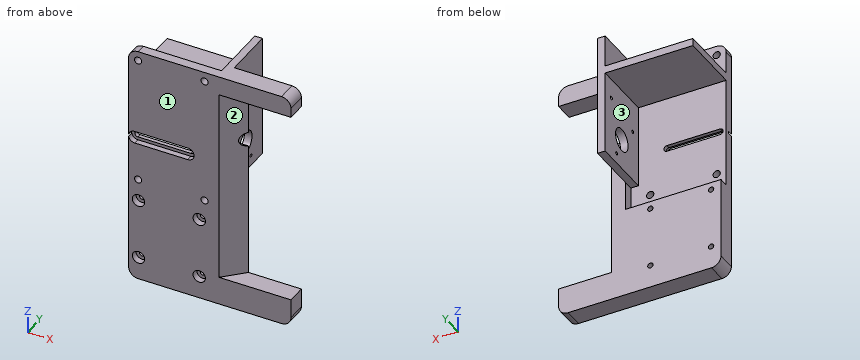
Autodesk Inventor part; units mm, degrees
ref_plane "Arbeitsebene4" through (-41.55, 10, -74.35) normal (0, -1, 0) x (1, 0, 0)
ref_plane "Arbeitsebene5" through (-44.55, 5, -0.85) normal (0, -1, 0) x (1, 0, 0)
ref_plane "Arbeitsebene7" through (7.45, -0.1921, -3.518) normal (-1, 0, 0) x (0, -0.417504, 0.9086751)
ref_plane "Arbeitsebene4" through (-41.55, 10, -74.35) normal (0, -1, 0) x (1, 0, 0)
sketch "Skizze1" plane through (0, 0, 0) normal (0, 1, 0) x (-1, 0, 0)
  line L0 (-37.75, -63.9) -> (37.75, -63.9)
  line L1 (42.75, -58.9) -> (42.75, 58.9)
  line L2 (37.75, 63.9) -> (-37.75, 63.9)
  line L3 (-42.75, 58.9) -> (-42.75, -58.9)
  line L4 (-42.75, -63.9) -> (42.75, 63.9) construction
  line L5 (42.75, -63.9) -> (-42.75, 63.9) construction
  arc A0 (42.75, 58.9) -> (37.75, 63.9) centre (37.75, 58.9) ccw
  arc A1 (-37.75, 63.9) -> (-42.75, 58.9) centre (-37.75, 58.9) ccw
  arc A2 (-42.75, -58.9) -> (-37.75, -63.9) centre (-37.75, -58.9) ccw
  arc A3 (37.75, -63.9) -> (42.75, -58.9) centre (37.75, -58.9) ccw
  point P0 (0, 0)
  dimension "d0" = 85.5
  dimension "d1" = 127.8
  dimension "d2" = 5
extrude "Extrusion1" add sketch "Skizze1" along normal up to surface (10 mm away)
ref_plane "Arbeitsebene1" through (37.75, 0, 0) normal (0, 0, -1) x (-1, 0, 0)
ref_plane "Arbeitsebene2" through (0, 0, 58.9) normal (1, 0, 0) x (0, 0, -1)
sketch "Skizze10" plane through (0, 0, 0) normal (0, -1, 0) x (1, 0, 0)
  circle A0 centre (-37.55, -51.85) radius 1.75
  circle A1 centre (-37.55, -19.85) radius 1.75
  circle A2 centre (-5.55, -51.85) radius 1.75
  circle A3 centre (-5.55, -19.85) radius 1.75
  circle A4 centre (-37.55, -51.85) radius 1.4
  point P0 (0, 0)
  dimension "d37" = 2.8
hole "Bohrung2" at (-37.55, 0, -51.85) at (-37.55, 0, -19.85) at (-5.55, 0, -19.85) at (-5.55, 0, -51.85) direction (0, 1, 0) diameter 2.8 end through all counterbore diameter 6.5 counterbore depth 3.5
sketch "Skizze11" plane through (-37.75, 10, -63.9) normal (0, 1, 0) x (1, 0, 0)
  line L0 (-6.8, -63.05) -> (41.2, -63.05)
  line L1 (-6.8, -95.05) -> (41.2, -95.05)
  line L2 (-3.8, -48.05) -> (36.2, -48.05)
  line L3 (-5, -5) -> (-5, -122.8)
  line L4 (0, -127.8) -> (75.5, -127.8)
  line L5 (-5, -48.05) -> (45.2, -48.05)
  line L6 (45.2, -48.05) -> (45.2, -127.8)
  line L7 (45.2, -127.8) -> (-5, -127.8)
  line L8 (-5, -127.8) -> (-5, -48.05)
  line L9 (45.2, -108.7984) -> (45.2, -60.5539)
  line L10 (80.5, -82.3) -> (60.5, -82.3) construction
  line L11 (60.5, -82.3) -> (60.5, -82.05) construction
  line L12 (60.5, -82.05) -> (60.5, -81.8) construction
  line L13 (60.5, -81.8) -> (60.5, -81.55) construction
  line L14 (60.5, -81.55) -> (60.5, -81.3) construction
  line L15 (60.5, -81.3) -> (60.5, -81.05) construction
  line L16 (60.5, -81.05) -> (60.5, -80.8) construction
  line L17 (60.5, -80.8) -> (60.5, -80.55) construction
  line L18 (60.5, -80.55) -> (60.5, -80.3) construction
  line L19 (60.5, -80.3) -> (60.5, -80.05) construction
  line L20 (60.5, -80.05) -> (60.5, -79.8) construction
  line L21 (60.5, -79.8) -> (60.5, -79.55) construction
  line L22 (60.5, -79.55) -> (60.5, -79.3) construction
  line L23 (60.5, -79.3) -> (60.5, -79.05) construction
  line L24 (60.5, -79.05) -> (60.5, -78.8) construction
  line L25 (60.5, -78.8) -> (60.5, -78.55) construction
  line L26 (60.5, -78.55) -> (60.5, -78.3) construction
  line L27 (60.5, -78.3) -> (60.5, -78.05) construction
  line L28 (60.5, -78.05) -> (60.5, -77.8) construction
  line L29 (60.5, -77.8) -> (60.5, -77.55) construction
  line L30 (60.5, -77.55) -> (60.5, -77.3) construction
  line L31 (60.5, -77.3) -> (80.5, -77.3) construction
  line L32 (80.5, -77.3) -> (80.5, -41.8) construction
  line L33 (80.5, -41.8) -> (54.7, -41.8) construction
  line L34 (54.7, -41.8) -> (54.7, -117.8) construction
  line L35 (54.7, -117.8) -> (80.5, -117.8) construction
  line L36 (80.5, -117.8) -> (80.5, -82.3) construction
  point P0 (37.75, -63.9)
  dimension "d45" = 0
ref_plane "Arbeitsebene5" through (-44.55, 5, -0.85) normal (0, -1, 0) x (1, 0, 0)
extrude "Extrusion9" cut sketch "Skizze11" against normal up to surface (5 mm away)
sketch "Skizze12" plane through (0, 0, 0) normal (0, -1, 0) x (1, 0, 0)
  circle A0 centre (-39.55, 15.15) radius 1.4
  circle A1 centre (-11.55, 15.15) radius 1.4
  line L0 (-11.55, 15.15) -> (-39.55, 15.15) construction
  line L1 (-11.55, 16.75) -> (-39.55, 16.75)
  line L2 (-39.55, 13.55) -> (-11.55, 13.55)
  arc A2 (-11.55, 13.55) -> (-11.55, 16.75) centre (-11.55, 15.15) ccw
  arc A3 (-39.55, 16.75) -> (-39.55, 13.55) centre (-39.55, 15.15) ccw
  point P0 (0, 0)
  point P1 (-25.55, 15.15)
  dimension "d48" = 3.2
extrude "Extrusion10" cut sketch "Skizze12" against normal blind 10 contours A0 | A1 | A2 L2 A3 L1
sketch "Skizze13" plane through (0, 0, 0) normal (0, -1, 0) x (1, 0, 0)
  line L0 (-44.55, 31.15) -> (3.45, 31.15)
  line L1 (-11.55, 13.55) -> (-39.55, 13.55)
  arc A0 (-39.55, 16.75) -> (-39.55, 13.55) centre (-39.55, 15.15) ccw
  line L2 (-39.55, 16.75) -> (-11.55, 16.75)
  arc A1 (-11.55, 13.55) -> (-11.55, 16.75) centre (-11.55, 15.15) ccw
  arc A2 (-42.75, -58.9) -> (-37.75, -63.9) centre (-37.75, -58.9) ccw
  line L3 (37.75, -63.9) -> (-37.75, -63.9)
  arc A3 (37.75, -63.9) -> (42.75, -58.9) centre (37.75, -58.9) ccw
  line L4 (42.75, 58.9) -> (42.75, -58.9)
  arc A4 (42.75, 58.9) -> (37.75, 63.9) centre (37.75, 58.9) ccw
  line L5 (-37.75, 63.9) -> (37.75, 63.9)
  arc A5 (-37.75, 63.9) -> (-42.75, 58.9) centre (-37.75, 58.9) ccw
  line L6 (-42.75, -58.9) -> (-42.75, 58.9)
  line L7 (-11.55, 18.4) -> (-39.55, 18.4)
  arc A6 (-39.55, 18.4) -> (-39.55, 11.9) centre (-39.55, 15.15) ccw
  line L8 (-39.55, 11.9) -> (-11.55, 11.9)
  arc A7 (-11.55, 11.9) -> (-11.55, 18.4) centre (-11.55, 15.15) ccw
  point P0 (0, 0)
  dimension "d51" = 6.5
extrude "Extrusion11" cut sketch "Skizze13" against normal blind 3 contours L1 A0 L2 A1 | A6 L6 | L6 A6 L7 A7 L8
ref_plane "Arbeitsebene6" through (3.45, 21, 15.15) normal (1, 0, 0) x (0, 0, -1)
sketch "Skizze14" plane through (3.45, 21, 15.15) normal (1, 0, 0) x (0, 0, -1)
  line L0 (16, 16) -> (14, 16)
  line L1 (16, -16) -> (16, 16)
  line L2 (-16, 16) -> (-16, -16)
  circle A0 centre (-17.5, 10) radius 1 construction
  circle A1 centre (-11, -10.5) radius 1 construction
  line L3 (9.4, -16) -> (6.6, -16)
  circle A2 centre (10.5, 5) radius 1 construction
  circle A3 centre (0, 0) radius 6
  line L4 (-48.75, -21) -> (-48.75, -11)
  line L5 (16, 16) -> (-48.75, 16)
  line L6 (-48.75, 16) -> (-48.75, -16)
  line L7 (-48.75, -16) -> (16, -16)
  line L8 (16, -16) -> (16, 16)
  circle A4 centre (-17.5, 10) radius 0.9
  circle A5 centre (10.5, 5) radius 0.85
  circle A6 centre (-11, -10.5) radius 0.85
  point P0 (15.15, -21)
  point P1 (9.4, -16)
  point P2 (16, -16)
  point P3 (14, 16)
  point P4 (-48.75, -11)
  point P5 (6.6, -16)
  dimension "d56" = 1.8
  dimension "d57" = 1.7
  dimension "d58" = 1.7
ref_plane "Arbeitsebene7" through (7.45, -0.1921, -3.518) normal (-1, 0, 0) x (0, -0.417504, 0.9086751)
extrude "Extrusion12" add sketch "Skizze14" along normal up to surface (4 mm away)
sketch "Skizze15" plane through (-37.75, 10, -63.9) normal (0, 1, 0) x (1, 0, 0)
  line L0 (-5, -48.05) -> (45.2, -48.05)
  line L1 (45.2, -48.05) -> (45.2, -63.05)
  line L2 (45.2, -63.05) -> (45.2, -89.3626)
  line L3 (45.2, -89.3626) -> (45.2, -90.7374)
  line L4 (45.2, -90.7374) -> (45.2, -127.8)
  line L5 (45.2, -127.8) -> (75.5, -127.8)
  arc A0 (75.5, -127.8) -> (80.5, -122.8) centre (75.5, -122.8) ccw
  line L6 (80.5, -122.8) -> (80.5, -5)
  arc A1 (80.5, -5) -> (75.5, 0) centre (75.5, -5) ccw
  line L7 (75.5, 0) -> (0, 0)
  arc A2 (0, 0) -> (-5, -5) centre (0, -5) ccw
  line L8 (-5, -5) -> (-5, -48.05)
  line L9 (80.5, -117.8) -> (52.5869, -117.8)
  line L10 (52.5869, -117.8) -> (52.5869, -15)
  line L11 (52.5869, -15) -> (80.5, -15)
  line L12 (80.5, -15) -> (80.5, -117.8)
  line L13 (45.7, -42.1725) -> (45.7, -1.05)
  point P0 (37.75, -63.9)
  point P1 (80.5, -15)
  dimension "d59" = 10
  dimension "d60" = 15
extrude "Extrusion13" cut sketch "Skizze15" against normal through all contours L6 L9 L10 L11
sketch "Skizze16" plane through (7.45, 10, -0.85) normal (1, 0, 0) x (0, 0, -1)
  circle A0 centre (-27, 0.5) radius 1
  circle A1 centre (-27, 0.5) radius 0.85
  circle A2 centre (-27, 0.5) radius 3.8399
  point P0 (-0.85, -10)
extrude "Extrusion14" cut sketch "Skizze16" along normal up to surface (7.3869 mm away) contours A0 | A1 | A2
chamfer "Fase1" distance 10 angle 45 1 edges at (14.8369, 0, 2.5)
sketch "Skizze17" plane through (-42.75, 5, -15.85) normal (0, 1, 0) x (1, 0, 0)
  line L0 (46.2, -79.75) -> (46.2, -15)
  line L1 (46.2, -15) -> (50.2, -15)
  line L2 (50.2, -15) -> (50.2, 0)
  line L3 (50.2, 0) -> (0, 0)
  line L4 (0, -74.75) -> (0, 0)
  arc A0 (0, -74.75) -> (5, -79.75) centre (5, -74.75) ccw
  line L5 (46.2, -79.75) -> (5, -79.75)
  line L6 (3.2, -29.4) -> (31.2, -29.4)
  arc A1 (31.2, -32.6) -> (31.2, -29.4) centre (31.2, -31) ccw
  line L7 (31.2, -32.6) -> (3.2, -32.6)
  arc A2 (3.2, -29.4) -> (3.2, -32.6) centre (3.2, -31) ccw
  line L8 (5, -74.75) -> (40, -74.75)
  line L9 (40, -74.75) -> (40, -7.75)
  line L10 (40, -7.75) -> (5, -7.75)
  line L11 (5, -7.75) -> (5, -74.75)
  point P0 (42.75, -15.85)
  dimension "d68" = 35
  dimension "d69" = 67
hole "Bohrung3" at (-37.75, 5, -8.1) at (-2.75, 5, -8.1) at (-2.75, 5, 58.9) at (-37.75, 5, 58.9) direction (0, -1, 0) diameter 3.8 end through all
sketch "Skizze18" plane through (3.45, 37, 63.9) normal (0, 1, 0) x (1, 0, 0)
  line L0 (4, 64.75) -> (4, 0)
  line L1 (0, 64.75) -> (4, 64.75)
  line L2 (0, 64.75) -> (0, 0)
  line L3 (0, 0) -> (4, 0)
  line L4 (-46.2, 5) -> (-46.2, 79.75)
  line L5 (0, 16.8478) -> (-46.2, 16.8478)
  line L6 (-46.2, 16.8478) -> (-46.2, 20.8478)
  line L7 (-46.2, 20.8478) -> (0, 20.8478)
  line L8 (0, 20.8478) -> (0, 16.8478)
  point P0 (-3.45, 63.9)
  point P1 (0, 20.8478)
  point P2 (-46.2, 16.8478)
  dimension "d77" = 4
extrude "Extrusion15" add sketch "Skizze18" against normal up to surface (32 mm away) contours L2 L5 L4 L7
properties part number "TIRFImager_base_xyz_v0"
Input: part model. Units: mm. Frame: model coordinates. Face numbers are marked on the shaded views. Coordinates: 2 decimals unless noted, no trailing zeros. Loops run counter-clockwise (first coordinate to the right, second up) from the corner with the lowest first, then second, coordinate; pieces in that order, holes last.
Q1. Contact query for flat-ended pins moving along their axis: pin 1 (10 mm diameter, centred on x = -32.5, y = 26.5, fed in from -Z); pin 2 (10.5 mm diameter, centred on x = -5.55, z = -19.85, fed in from +Y); pin 3 (6 mm diameter, centred on x = -37.55, z = -19.85, fed in from -Y). Output: stop coordinate, or through.
Q2. Cut plane B-B (x = 20). Output: boundary loops of the cut face in (y, z), then the cut area to 3 significant figures.
Q3. Draft query along Z for the marked faces 1, 2 and 3. Return one class per face: +Z half, -Z half, draft (parallel to the pull), parting line (faces both ways), or undercut.
Q4. Cut plane C-C (z = 55.5). Output: boundary loops of the cut face in (x, y).
Q5. Cut plane A-A (z = -51.85). Output: boundary loops of the cut face in (x, y), then the cut area to 3 significant figures.
Q6. Material intervals for line 1 (Z direction, x = -37.55, y = 5.5); line 2 (X direction, y = 1.35, z = 58.9); line 3 (Z direction, x = -37.55, y = 1.15), sorted ascending.
Q7. Cut plane D-D (y = 13.5). Output: boundary loops of the cut face in (x, z).
Working result:
1. pin 1: stops at z = 43.05
1. pin 2: stops at y = 10
1. pin 3: stops at y = 3.5
2. outline: (0, -63.9) - (10, -63.9) - (10, -48.9) - (0, -48.9) - close; (0, 53.9) - (10, 53.9) - (10, 63.9) - (0, 63.9) - close
2. area: 250 mm2
3. face 1: draft
3. face 2: undercut
3. face 3: undercut
4. outline: (-42.75, 0) - (42.75, 0) - (42.75, 10) - (7.45, 10) - (7.45, 37) - (3.45, 37) - (3.45, 5) - (-42.75, 5) - close
5. outline: (-42.75, 0) - (-40.8, 0) - (-40.8, 3.5) - (-38.95, 3.5) - (-38.95, 10) - (-42.75, 10) - close; (-36.15, 3.5) - (-34.3, 3.5) - (-34.3, 0) - (-8.8, 0) - (-8.8, 3.5) - (-6.95, 3.5) - (-6.95, 10) - (-36.15, 10) - close; (-4.15, 3.5) - (-2.3, 3.5) - (-2.3, 0) - (42.75, 0) - (42.75, 10) - (-4.15, 10) - close
5. area: 773 mm2
6. line 1: z = -63.9 to -53.25, -50.45 to -21.25, -18.45 to -15.85, 43.05 to 47.05
6. line 2: x = -42.75 to -39.65, -35.85 to -4.65, -0.85 to 42.75
6. line 3: z = -63.9 to -55.1, -48.6 to -23.1, -16.6 to -9.99, -6.21 to 11.9, 18.4 to 57.01, 60.79 to 63.9
7. outline: (-42.75, 43.05) - (3.45, 43.05) - (3.45, -0.85) - (7.45, -0.85) - (7.45, 63.9) - (3.45, 63.9) - (3.45, 47.05) - (-42.75, 47.05) - close
